Verification items for this drawing (mm, ordinates from the low corner). A direction names the side the tool comes from. Coordinates: 2 decimals unless noted, no trailing zeros. Order: outer loops, then holes, each group sorted by start corner. A loop starts at its lowest first (then second) coordinate and runs counter-clockwise, first axis right, second up.
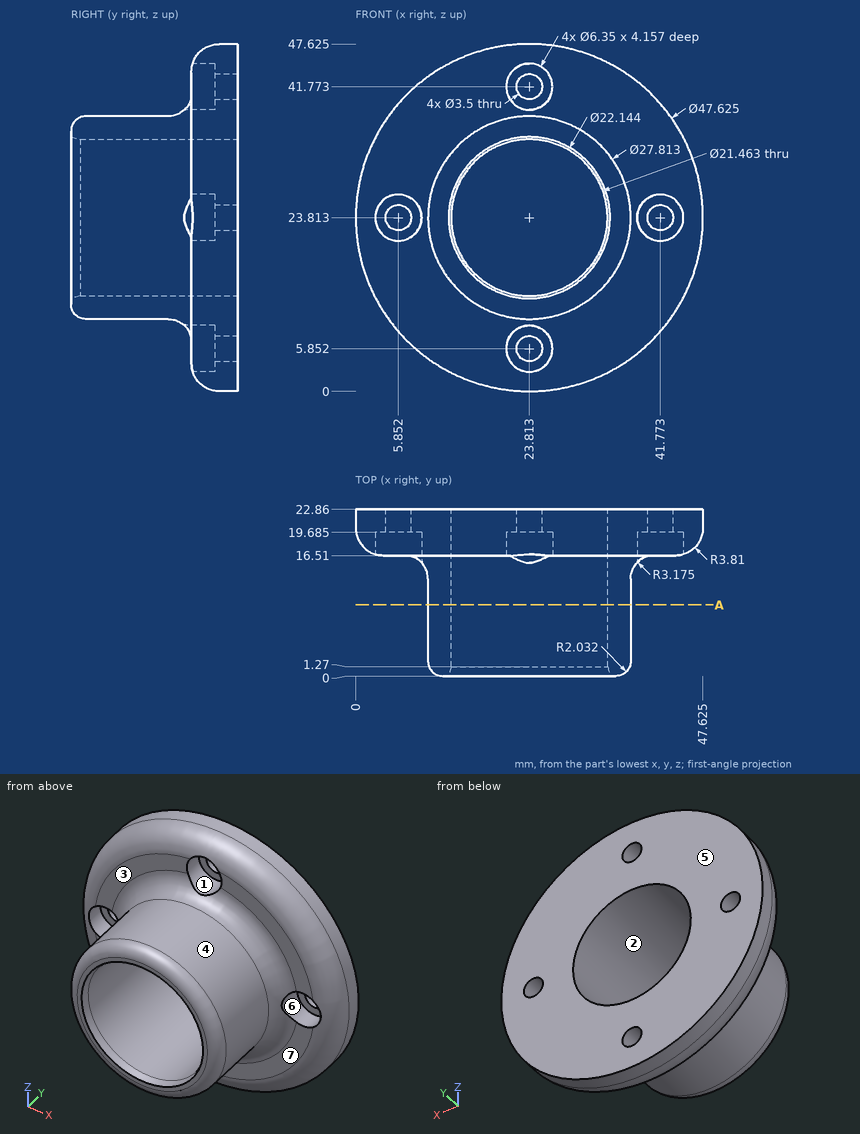
(1) Release check for a two-part mould opening along X. For the marked faces 1, 2, 3 and 4 record: +X half, -X half, draft (parallel to the pull), parting line (faces both ways), or undercut.
Filled in:
face 1: undercut
face 2: undercut
face 3: draft
face 4: parting line
(2) Thickness scan on probe 1 along Y at (x, z) = (22, 4) (1 decimal); probe 2 along X at (y, z) = (21.25, 23) (1 decimal); probe 3 along Z at (x, y) = (23.5, 19.25) (1 decimal). Record the ranges inside material, lowest first.
Filled in:
probe 1: y = 19.7 to 22.9
probe 2: x = 0 to 4.3, 7.4 to 13.1, 34.5 to 40.2, 43.3 to 47.6
probe 3: z = 0.2 to 2.7, 9 to 13.1, 34.5 to 38.6, 44.9 to 47.5
(3) Cross-section at A-A (y = 9.75). Enter the section's corners in (x, z) (1 decimal), and give its area (3 significant figures).
Filled in:
outline: circle Ø27.8 at (23.8, 23.8); hole circle Ø21.5 at (23.8, 23.8)
area: 246 mm2
(4) Tool access check on the marked faces 5, 6 and 7. Record the directions out of +Z, -Z, +X, -X, +Y, -Y that give a thin tool (end or side, any length) a straight path to the whole face; none if there is none.
Filled in:
face 5: +Z, -Z, +X, -X, +Y
face 6: -Y
face 7: -Z, +X, -Y
(5) Go/stop test with flat-tipped pins: P1, Ø7, axis at x = 41.5, z = 24, coming from the -Y side (1 decimal); P2, Ø1.5, axis at x = 17.5, z = 41.5, coming from the -Y side; P3, Ø3, axis at y = 16.5, z = 28, coming from the -X side. Record where each tip stops, or that it passes through.
Filled in:
P1: stops at y = 14.6
P2: stops at y = 16.51
P3: stops at x = 1.14
